Verification items for the finished model (mm, model axes). Face numbers are marked on the shaded views. Round coordinates to 2 decimals unless told otherwise and drop trailing zeros. Order: outer loops, then holes, each group sorted by start corner. A loop starts at its lowest first (then second) coordinate and runs counter-clockwise, first axis right, second up. Notation, with made-up numbers: M 41.25,2 L 95.25,2 A25 cw 95.25,17 Z; hole C -28,18 d3. An arc over 180 degrees is marked long. Write item = value, one per line. Start each with the question number.
from build123d import *

# Parameters (mm, degrees)
SKETCH1_W           = 97.90721761
SKETCH1_H           = 46.600763908
BOSS_EXTRUDE1_DEPTH = 20
CUT_EXTRUDE1_DEPTH  = 90
CUT_EXTRUDE3_DEPTH  = 90


with BuildPart() as part:
    # Sketch1 → Boss-Extrude1 (new body)
    with BuildSketch(Plane(origin=(0, 0, 0), x_dir=(1, 0, 0), z_dir=(0, 1, 0))):
        Rectangle(SKETCH1_W, SKETCH1_H)
    extrude(amount=BOSS_EXTRUDE1_DEPTH)

    # Sketch3 → Cut-Extrude1 (cut)
    with BuildSketch(Plane.ZY.offset(48.953608805)):
        Polygon((0, 10), (-10.601673789, 14.55), (-17.105, 14.55), (-17.105, 5.45), (-10.601673789, 5.45), align=None)
        Polygon((10.601673789, 14.55), (-10.601673789, 14.55), (0, 10), align=None)
        Polygon((10.601673789, 5.45), (0, 10), (-10.601673789, 5.45), align=None)
        Polygon((10.601673789, 14.55), (0, 10), (10.601673789, 5.45), (17.105, 5.45), (17.105, 14.55), align=None)
    extrude(amount=-CUT_EXTRUDE1_DEPTH, mode=Mode.SUBTRACT)

    # Sketch4 → Cut-Extrude3 (cut)
    with BuildSketch(Plane.ZY.offset(48.953608805)):
        Polygon((-14.105, 4.45), (-14.105, 2.45), (14.105, 2.45), (14.105, 4.45), (17.955, 4.45), (17.955, 14.55), (17.105, 14.55), (17.105, 5.45), (-17.105, 5.45), (-17.105, 14.55), (-17.955, 14.55), (-17.955, 4.45), align=None)
    extrude(amount=-CUT_EXTRUDE3_DEPTH, mode=Mode.SUBTRACT)


solid = part.part
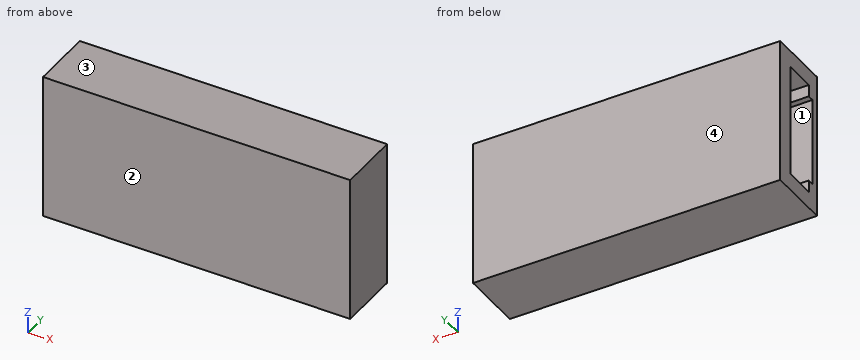
1) Release check for a two-part mould opening along Y. For the marked faces 1, 2, 3 and 4 record: pulls with the +Y half, pulls with the -Y half, needs draft (parallel to the pull), parting line crosses it, or undercut.
2) Scan lines: probe 1 along Z at (x, y) = (-25, 9.25) (3 decimals); probe 2 along Y at (x, z) = (-13, -13); probe 3 along Y at (x, z) = (-21.5, -16). Record each from-to range of solid material in increasing order.
3) Gauge pin test, flat end, axial feed: P1, Ø1, axis at y = 4, z = -3, coming from the -X side. Record the tip position at first contact, or that the pin passes through.
4) Cross-section at C-C, the plane z = 0. Enter the section's corners in (x, y), then the cut area to 3 significant figures.
5) Cross-section at A-A, the plane x = -33. Enter the section's corners in (y, z) (3 decimals), then the cut area to 3 significant figures.
6) Cross-section at B-B, the plane y = 7.75. Enter the section's corners in (x, z) (3 decimals), then the cut area to 3 significant figures.
Geometry results:
q1.face_1 = undercut
q1.face_2 = pulls with the -Y half
q1.face_3 = needs draft
q1.face_4 = pulls with the +Y half
q2.probe_1 = -23.3 to -17.955, 17.955 to 23.3
q2.probe_2 = 0 to 2.45, 14.55 to 20
q2.probe_3 = 0 to 4.45, 14.55 to 20
q3.P1 = 41.05
q4.outline = M -48.95,0 L 48.95,0 L 48.95,20 L -48.95,20 L -48.95,14.55 L 41.05,14.55 L 41.05,2.45 L -48.95,2.45 Z
q4.area = 869 mm^2
q5.outline = M 0,-23.3 L 20,-23.3 L 20,23.3 L 0,23.3 Z; hole M 2.45,-14.105 L 4.45,-14.105 L 4.45,-17.955 L 14.55,-17.955 L 14.55,17.955 L 4.45,17.955 L 4.45,14.105 L 2.45,14.105 Z
q5.area = 513 mm^2
q6.outline = M -48.954,-23.3 L 48.954,-23.3 L 48.954,23.3 L -48.954,23.3 L -48.954,17.955 L 41.046,17.955 L 41.046,-17.955 L -48.954,-17.955 Z
q6.area = 1,330 mm^2
